Model file for the job. Use its own axes, mm. Round coordinates to 2 decimals unless told otherwise and drop trailing zeros. Order: outer loops, then holes, each group sorted by start corner. A loop starts at its lowest first (then second) coordinate and runs counter-clockwise, first axis right, second up. Notation, with made-up numbers: (17.25, 41.5) - (51.25, 41.5) arc R15 cw to (51.25, 69.5) - close; hole circle Ø11 at (42, -25.75). An arc over 180 degrees is marked (long way). Put each result on its own line as item: value. Start each with the question number.
Item 1: Saw through at A-A on y = 0. List the corners of the cut face in (x, z) (3 decimals), plus the area to 3 significant figures.
Item 2: Saw through at C-C on x = 11.5. List the corners of the cut face in (y, z) (3 decimals).
Item 3: Pin check, flat tips, straight feed: pin 1 Ø1 at (x, y) = (2, 8.5) entering from -Z; pin 2 Ø1 at (x, z) = (4, -13.5) entering from -Y; pin 3 Ø3 at (x, z) = (4, 13) entering from -Y. Stop position of each tip, or through.
Item 4: Mould opens along Z. For faces 1 (the face through (2.119, 7.925, 15.237)), 2 (the face through (15, 7.6, -11.4)), 3 (the face through (7.591, 11.923, 3.755)) say: pulls with the +Z half, pulls with the -Z half, needs draft (parallel to the pull), parting line crosses it, or undercut.
Item 5: Probe probe 1 along Z at (x, y) = (3.5, 0) (3 decimals); probe 2 along Z at (x, y) = (14, 7); probe 3 along Y at (x, z) = (2, -8). List the from-to ranges inside material, lowest first.
Autodesk Inventor part; units mm, degrees
ref_plane "YZ Plane" through (0, 0, 0) normal (1, 0, 0) x (0, 1, 0)
ref_plane "XZ Plane" through (0, 0, 0) normal (0, 1, 0) x (-1, 0, 0)
ref_plane "XY Plane" through (0, 0, 0) normal (0, 0, 1) x (1, 0, 0)
sketch "Sketch_1" plane through (0, 0, 0) normal (0, 0, 1) x (1, 0, 0)
  line L0 (50, 0) -> (-50, 0)
  arc A0 (0, 13.5) -> (1, 12.5) centre (1, 13.5) ccw
  line L1 (1, 12.5) -> (14, 12.5)
  arc A1 (14, 12.5) -> (15, 13.5) centre (14, 13.5) ccw
  line L2 (15, 13.5) -> (15, 17.175)
  line L3 (15, 17.175) -> (10.7022, 17.175)
  arc A2 (4.2978, 17.175) -> (10.7022, 17.175) centre (7.5, 19.52) ccw
  line L4 (4.2978, 17.175) -> (0, 17.175)
  line L5 (0, 17.175) -> (0, 13.5)
revolve "Revolution1" add sketch "Sketch_1" angle 360 about axis through (50, 0, 0) along (1, 0, 0)
properties part number "6205_PART1"
Results found:
1. outline: (0, -17.175) - (4.298, -17.175) arc R3.969 cw to (10.702, -17.175) - (15, -17.175) - (15, -13.5) arc R1 ccw to (14, -12.5) - (1, -12.5) arc R1 ccw to (0, -13.5) - close; (0, 13.5) arc R1 ccw to (1, 12.5) - (14, 12.5) arc R1 ccw to (15, 13.5) - (15, 17.175) - (10.702, 17.175) arc R3.969 cw to (4.298, 17.175) - (0, 17.175) - close
1. area: 125 mm²
2. outline: circle Ø34.35 at (0, 0); hole circle Ø25 at (0, 0)
3. pin 1: stops at z = -15.2
3. pin 2: stops at y = -11.22
3. pin 3: stops at y = -12.76
4. face 1: parting line crosses it
4. face 2: needs draft
4. face 3: undercut
5. probe 1: z = -17.175 to -12.5, 12.5 to 17.175
5. probe 2: z = -15.68 to -10.36, 10.36 to 15.68
5. probe 3: y = -15.2 to -9.6, 9.6 to 15.2
